```python
from build123d import *

# Parameters (mm, degrees)
F0_W     = 100
F0_H     = 100
F1_DEPTH = 19
F2_R     = 12.081431
F3_DEPTH = 19
F4_R     = 10.963325
F5_DEPTH = 19
F6_R     = 10
F7_DEPTH = 19


with BuildPart() as f1:
    # F0 (on Top) → F1 (new body)
    with BuildSketch(Plane.XY):
        with Locations((-35.732688, -12.833619)):
            Rectangle(F0_W, F0_H)
    extrude(amount=F1_DEPTH)

    # F2 (on face) → F3 (cut)
    with BuildSketch(Plane.XY.offset(19)):
        with Locations((-59.289314, 9.998217)):
            Circle(F2_R)
    extrude(amount=-F3_DEPTH, mode=Mode.SUBTRACT)

    # F4 (on face) → F5 (cut)
    with BuildSketch(Plane.XY.offset(19)):
        with Locations((-11.882036, 11.570971)):
            Circle(F4_R)
    extrude(amount=-F5_DEPTH, mode=Mode.SUBTRACT)

    # F6 (on face) → F7 (cut)
    with BuildSketch(Plane.XY.offset(19)):
        with Locations((-64.806127, -28.333058)):
            Circle(F6_R)
        with Locations((-20.744683, -26.488627)):
            Circle(F6_R)
    extrude(amount=-F7_DEPTH, mode=Mode.SUBTRACT)


solid = f1.part
```
Here's how the part is built. I have some questions about the finished solid (model axes, mm). Round coordinates to 2 decimals unless told otherwise and drop trailing zeros. Order: outer loops, then holes, each group sorted by start corner. A loop starts at its lowest first (then second) coordinate and runs counter-clockwise, first axis right, second up. Notation, with made-up numbers: (-26, -5.75) -> (28, -5.75) arc R18 ccw to (28, 16.25) -> close; hole circle Ø9 at (-26, 54.25). An arc over 180 degrees is marked (long way). Use a Markdown table: item, result. Add a question column.
(1) Suppose I cut it at D-D, the plane z = 16.75. Please give me the cut outline in (x, y).
(2) If we mould it in two halves opening along X, with no side actions, what happens to faces 1 (the face through (-85.733, -14, 9)), 2 (the face through (14.267, -14, 9)), 3 (the face through (-14.26, 0.87, 9.63))? For each: released by +X, released by -X, zero draft, split by the parting line, or undercut.
(3) I need wall thicknesses on line 1 along X through (y, z) = (19.5, 9.5); line 2 along X through (y, z) = (12.5, 15.25); line 3 along Y through (x, z) = (-22, 15.5). Which ranges of each line are inside material? Lowest first, please.
(4) Suppose I cut it at A-A, the plane x = -69.5. Please give me the cut outline in (y, z).
(5) Suppose I cut it at B-B, the plane y = 13. Please give me the cut outline in (x, z), and give its area (3 significant figures).
(6) Suppose I cut it at C-C, the plane x = -6. Please give me the cut outline in (y, z), and give its area (3 significant figures).
Verdict:
| question | item | result |
|---|---|---|
| 1 | outline | (-85.73, -62.83) -> (14.27, -62.83) -> (14.27, 37.17) -> (-85.73, 37.17) -> close; hole circle Ø20 at (-64.81, -28.33); hole circle Ø24.16 at (-59.29, 10); hole circle Ø20 at (-20.74, -26.49); hole circle Ø21.93 at (-11.88, 11.57) |
| 2 | face 1 | released by -X |
| 2 | face 2 | released by +X |
| 2 | face 3 | undercut |
| 3 | line 1 | -85.73 to -66.75, -51.83 to -19.45, -4.31 to 14.27 |
| 3 | line 2 | -85.73 to -71.11, -47.47 to -22.81, -0.96 to 14.27 |
| 3 | line 3 | -62.83 to -36.41, -16.57 to 7.35, 15.79 to 37.17 |
| 4 | outline | (-62.83, 0) -> (-37.16, 0) -> (-37.16, 19) -> (-62.83, 19) -> close; (-19.5, 0) -> (3.54, 0) -> (3.54, 19) -> (-19.5, 19) -> close; (16.46, 0) -> (37.17, 0) -> (37.17, 19) -> (16.46, 19) -> close |
| 5 | outline | (-85.73, 0) -> (-70.99, 0) -> (-70.99, 19) -> (-85.73, 19) -> close; (-47.59, 0) -> (-22.75, 0) -> (-22.75, 19) -> (-47.59, 19) -> close; (-1.01, 0) -> (14.27, 0) -> (14.27, 19) -> (-1.01, 19) -> close |
| 5 | area | 1,040 mm2 |
| 6 | outline | (-62.83, 0) -> (2.32, 0) -> (2.32, 19) -> (-62.83, 19) -> close; (20.82, 0) -> (37.17, 0) -> (37.17, 19) -> (20.82, 19) -> close |
| 6 | area | 1,550 mm2 |
